Can you work these out from the model? Positions are in its coordinate system, mm. A direction names the side the tool comes from. Coordinates: 2 decimals unless noted, no trailing zeros. Order: outer loops, then holes, each group sorted by start corner. A loop starts at its lowest first (then second) coordinate and runs counter-clockwise, first axis right, second up. Notation, with made-up numbers: (83, 2) -> (123, 2) arc R27 ccw to (123, 34) -> close; hole circle Ø9 at (9, 88.5). An arc over 180 degrees is marked (long way). Answer in a Markdown table with one row per item.
```python
from build123d import *

# Parameters (mm, degrees)
SKETCH1_W           = 63.5
SKETCH1_H           = 127
SKETCH1_R           = 2
BOSS_EXTRUDE1_DEPTH = 6.35
SKETCH2_R           = 2
SKETCH2_W           = 6.35
SKETCH2_H           = 12.7
CUT_EXTRUDE1_DEPTH  = 6.35


with BuildPart() as part:
    # Sketch1 → Boss-Extrude1 (new body)
    with BuildSketch(Plane(origin=(0, 0, 0), x_dir=(1, 0, 0), z_dir=(0, 1, 0))):
        with Locations((31.75, 63.5)):
            Rectangle(SKETCH1_W, SKETCH1_H)
        with Locations((3.175, 12.7)):
            Circle(SKETCH1_R, mode=Mode.SUBTRACT)
        with Locations((60.325, 12.7)):
            Circle(SKETCH1_R, mode=Mode.SUBTRACT)
        with Locations((31.75, 60.325)):
            Circle(SKETCH1_R, mode=Mode.SUBTRACT)
    extrude(amount=BOSS_EXTRUDE1_DEPTH)

    # Sketch2 → Cut-Extrude1 (cut)
    with BuildSketch(Plane(origin=(0, 6.35, 0), x_dir=(1, 0, 0), z_dir=(0, 1, 0))):
        with Locations((34.925, 101.6)):
            Circle(SKETCH2_R)
        with Locations((34.925, 89.48002155)):
            Rectangle(SKETCH2_W, SKETCH2_H)
        with Locations((34.925, 114.88002155)):
            Rectangle(SKETCH2_W, SKETCH2_H)
    extrude(amount=-CUT_EXTRUDE1_DEPTH, mode=Mode.SUBTRACT)


solid = part.part
```
(1) We'd pull the mould along X, two halves only. Please class faces 1 (the flat face through (0, 3, -63)), 2 (the flat face through (31, 3, -127)), 3 (the flat face through (38.1, 3, -89)): +X half, -X half, draft (parallel to the pull), parting line (faces both ways), or undercut.
Response values:
| item | result |
|---|---|
| face 1 | -X half |
| face 2 | draft |
| face 3 | undercut |
(2) Suppose I cut it at B-B (z = -12.7). Please give me the cut outline in (x, y) (3 decimals).
Response values:
| item | result |
|---|---|
| outline | (0, 0) -> (1.175, 0) -> (1.175, 6.35) -> (0, 6.35) -> close; (5.175, 0) -> (58.325, 0) -> (58.325, 6.35) -> (5.175, 6.35) -> close; (62.325, 0) -> (63.5, 0) -> (63.5, 6.35) -> (62.325, 6.35) -> close |
(3) Suppose I cut it at C-C (y = 2.5). Please give me the cut outline in (x, z) (3 decimals), and give its area (3 significant figures).
Response values:
| item | result |
|---|---|
| outline | (0, -127) -> (63.5, -127) -> (63.5, 0) -> (0, 0) -> close; hole circle Ø4 at (3.175, -12.7); hole circle Ø4 at (31.75, -60.325); hole (31.75, -121.23) -> (38.1, -121.23) -> (38.1, -108.53) -> (31.75, -108.53) -> close; hole (31.75, -95.83) -> (38.1, -95.83) -> (38.1, -83.13) -> (31.75, -83.13) -> close; hole circle Ø4 at (34.925, -101.6); hole circle Ø4 at (60.325, -12.7) |
| area | 7,850 mm2 |
(4) Suppose I cut it at D-D (x = 35.5). Please give me the cut outline in (y, z).
Response values:
| item | result |
|---|---|
| outline | (0, -127) -> (6.35, -127) -> (6.35, -121.23) -> (0, -121.23) -> close; (0, -108.53) -> (6.35, -108.53) -> (6.35, -103.52) -> (0, -103.52) -> close; (0, -99.68) -> (6.35, -99.68) -> (6.35, -95.83) -> (0, -95.83) -> close; (0, -83.13) -> (6.35, -83.13) -> (6.35, 0) -> (0, 0) -> close |
(5) Suppose I cut it at A-A (z = -110). Please give me the cut outline in (x, y).
Response values:
| item | result |
|---|---|
| outline | (0, 0) -> (31.75, 0) -> (31.75, 6.35) -> (0, 6.35) -> close; (38.1, 0) -> (63.5, 0) -> (63.5, 6.35) -> (38.1, 6.35) -> close |
(6) Will this pin go through, and if not, where does the flat tip stop? pin 1 Ø3.5 at (x, z) = (34.925, -101.6) entering from -Y.
Response values:
| item | result |
|---|---|
| pin 1 | through |
(7) On a 3-axis mill with a long thin cutter (end or side, diameter ignored), from which of +Z, -Z, +X, -X, +Y, -Y can I reach the whole of each face in a straight line? I mean faces 4 (the flat face through (35, 3, -121.23)), 5 (the flat face through (31, 3, 0)). Say none if no direction works.
Response values:
| item | result |
|---|---|
| face 4 | +Y, -Y |
| face 5 | +Z, +X, -X, +Y, -Y |
(8) I need wall thicknesses on line 1 (Z direction, x = 37, y = 1.25); line 2 (X direction, y = 2.25, z = -12.7) (3 decimals); line 3 (X direction, y = 1, z = -14.5). Which ranges of each line are inside material? Lowest first, please. Write a range as [from, to].
Response values:
| item | result |
|---|---|
| line 1 | [-127, -121.23], [-108.53, -95.83], [-83.13, 0] |
| line 2 | [0, 1.175], [5.175, 58.325], [62.325, 63.5] |
| line 3 | [0, 2.3], [4.05, 59.45], [61.2, 63.5] |
